The listing builds one solid part. Answer for the finished solid, in the listing's coordinates (mm). Face numbers are marked on the shaded views. A direction names the side the tool comes from. Give positions to 0.01 mm unless a question says otherwise; leave off trailing zeros. Loops run counter-clockwise (first coordinate to the right, second up) from the corner with the lowest first, then second, coordinate; pieces in that order, holes last. Notation, with made-up numbers: M 43.5,-36.5 L 84.5,-36.5 A12 cw 84.5,-19.5 Z; hole C 28.5,-12.5 d9. An arc over 180 degrees is marked long. One line per item, written item: value. Start each with the question number.
Q1. A cutting plane is placed at C-C, the plane z = 1.5. Determine the outline of the cut face in (x, y).
Q2. For the marked faces 1 and 2, determine the directions among +Z, -Z, +X, -X, +Y, -Y from which every point of the face is accessible in a straight line to the end or side of a thin tool.
Q3. Consider L1, parallel to Z at x = 0.15, y = 0.4; L2, parallel to Z at x = 0.75, y = -2.1; L3, parallel to X at y = -0.2, z = 10. Determine where each line is inside the solid, lowest interval first.
Q4. Flat-ended cylindrical pins translate along their axes: pin 1 (2.5 mm diameter, centred on x = 0.5, y = 0.5, fed in from -Z); pin 2 (0.6 mm diameter, centred on y = 1, z = 0.5, fed in from -X); pin 3 (0.6 mm diameter, centred on y = 0.5, z = 0, fed in from +X); pin 4 (2 mm diameter, centred on x = 0, z = 1.5, fed in from -Y). Find the tip coordinate at first contact, or state that the pin passes through.
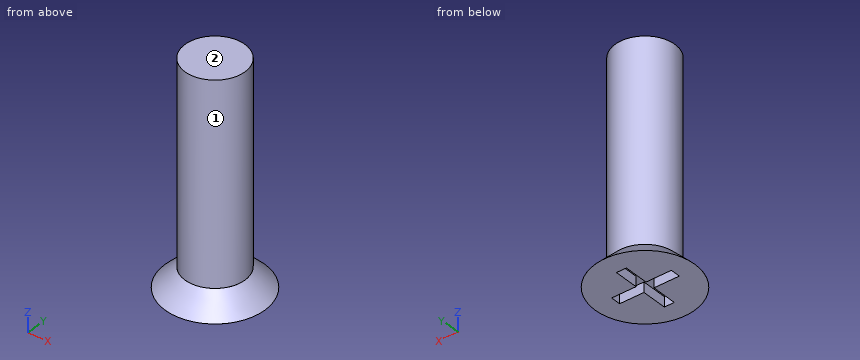
Autodesk Inventor part; units mm, degrees
ref_plane "YZ Plane" through (0, 0, 0) normal (1, 0, 0) x (0, 1, 0)
ref_plane "XZ Plane" through (0, 0, 0) normal (0, 1, 0) x (-1, 0, 0)
ref_plane "XY Plane" through (0, 0, 0) normal (0, 0, 1) x (1, 0, 0)
sketch "Sketch1" plane through (0, 0, 0) normal (0, 0, 1) x (1, 0, 0)
  circle A0 centre (0, 0) radius 2.5
  circle A1 centre (0, 0) radius 1.5
  dimension "d0" = 5
  dimension "d1" = 3
extrude "Extrusion1" add sketch "Sketch1" along normal blind 1
extrude "Extrusion2" add sketch "Sketch1" along normal blind 11 contours A1
chamfer "Chamfer1" distance 1 angle 45 1 edges at (-2.5, 0, 1)
sketch "Sketch2" plane through (0, 0, 0) normal (0, 0, -1) x (-1, 0, 0)
  circle A0 centre (0, 0) radius 2.5
  line L0 (0.25, -1.5229) -> (-0.25, -1.5229)
  line L1 (-0.25, 1.4771) -> (0.25, 1.4771)
  line L2 (0.25, -1.4771) -> (-0.25, 1.4771) construction
  line L3 (1.5229, 0.25) -> (1.5229, -0.25)
  line L4 (-1.4771, -0.25) -> (-1.4771, 0.25)
  line L5 (1.4771, 0.25) -> (-1.4771, -0.25) construction
  line L6 (1.5229, -0.25) -> (0.25, -0.25)
  line L7 (-0.25, -0.25) -> (-1.4771, -0.25)
  line L8 (-1.4771, 0.25) -> (-0.25, 0.25)
  line L9 (0.25, 0.25) -> (1.5229, 0.25)
  line L10 (0.25, 1.4771) -> (0.25, 0.25)
  line L11 (0.25, -0.25) -> (0.25, -1.5229)
  line L12 (-0.25, -1.5229) -> (-0.25, -0.25)
  line L13 (-0.25, 0.25) -> (-0.25, 1.4771)
  point P0 (-1.3278, 0)
  dimension "d9" = 0.5
  dimension "d10" = 3
  dimension "d11" = 0.5
  dimension "d12" = 3
extrude "Extrusion3" cut sketch "Sketch2" against normal blind 0.5 contours L0 L12 L7 L4 L8 L13 L1 L10 L9 L3 L6 L11
properties part number "Tornillo tapa"
Answer block:
1. outline: C 0,0 d3
2. face 1: +Z
2. face 2: +Z, +X, -X, +Y, -Y
3. L1: 0.5 to 11
3. L2: 0 to 0.27
3. L3: -1.49 to 1.49
4. pin 1: z = 0
4. pin 2: x = -2.1
4. pin 3: x = 2.49
4. pin 4: y = -2
